```python
from build123d import *

# Parameters (mm, degrees)
F1_DEPTH = 16.002
F3_DEPTH = 16.002
F4_R     = 2.54


with BuildPart() as f1:
    # F0 (on Top) → F1 (new body)
    with BuildSketch(Plane.XY):
        with BuildLine():
            ThreePointArc((38.1, -7.874), (48.1578868556, -3.7078868556), (52.324, 6.35))
            Line((52.324, 6.35), (52.324, 38.1))
            Line((52.324, 38.1), (-14.224, 38.1))
            Line((-14.224, 38.1), (-14.224, 6.35))
            ThreePointArc((-14.224, 6.35), (-10.0578868556, -3.7078868556), (0, -7.874))
            Line((0, -7.874), (38.1, -7.874))
        make_face()
        with BuildLine():
            Line((38.1, 0), (0, 0))
            ThreePointArc((0, 0), (-6.35, 6.35), (0, 12.7))
            Line((0, 12.7), (38.1, 12.7))
            ThreePointArc((38.1, 12.7), (44.45, 6.35), (38.1, 0))
        make_face(mode=Mode.SUBTRACT)
    extrude(amount=F1_DEPTH)

    # F2 (on face) → F3 (join)
    with BuildSketch(Plane(origin=(0, 38.1, 0), x_dir=(-1, 0, 0), z_dir=(0, 1, 0))):
        with BuildLine():
            Line((26.924, 0), (26.924, 44.45))
            Line((26.924, 44.45), (20.574, 44.45))
            ThreePointArc((20.574, 44.45), (14.224, 38.1), (7.874, 44.45))
            Line((7.874, 44.45), (1.524, 44.45))
            Line((1.524, 44.45), (1.524, 0))
            Line((1.524, 0), (26.924, 0))
        make_face()
        with BuildLine():
            Line((20.574, 44.45), (26.924, 44.45))
            ThreePointArc((26.924, 44.45), (14.224, 57.15), (1.524, 44.45))
            Line((1.524, 44.45), (7.874, 44.45))
            ThreePointArc((7.874, 44.45), (14.224, 50.8), (20.574, 44.45))
        make_face()
        with BuildLine():
            Line((-39.624, 0), (-39.624, 44.45))
            Line((-39.624, 44.45), (-45.974, 44.45))
            ThreePointArc((-45.974, 44.45), (-52.324, 38.1), (-58.674, 44.45))
            Line((-58.674, 44.45), (-65.024, 44.45))
            Line((-65.024, 44.45), (-65.024, 0))
            Line((-65.024, 0), (-39.624, 0))
        make_face()
        with BuildLine():
            Line((-45.974, 44.45), (-39.624, 44.45))
            ThreePointArc((-39.624, 44.45), (-52.324, 57.15), (-65.024, 44.45))
            Line((-65.024, 44.45), (-58.674, 44.45))
            ThreePointArc((-58.674, 44.45), (-52.324, 50.8), (-45.974, 44.45))
        make_face()
    extrude(amount=-F3_DEPTH)

    # F4
    f4_edges = [f1.edges().sort_by_distance(p)[0] for p in [
        (52.324, 14.224, 16.002),
        (-10.057887, -3.707887, 16.002),
        (-14.224, 14.224, 16.002),
        (-7.874, 22.098, 16.002),
        (-1.524, 30.099, 16.002),
        (19.05, 38.1, 16.002),
        (39.624, 30.099, 16.002),
        (45.974, 22.098, 16.002),
        (48.157887, -3.707887, 16.002),
        (19.05, -7.874, 16.002),
        (44.45, 6.35, 16.002),
        (19.05, 12.7, 16.002),
        (19.05, 0, 16.002),
        (-6.35, 6.35, 16.002),
        (52.324, 22.098, 8.001),
        (52.324, 38.1, 57.15),
        (65.024, 38.1, 22.225),
        (39.624, 38.1, 30.226),
        (-1.524, 38.1, 30.226),
        (-14.224, 38.1, 57.15),
        (-26.924, 38.1, 22.225),
        (-14.224, 22.098, 8.001),
    ]]
    fillet(f4_edges, radius=F4_R)


solid = f1.part
```
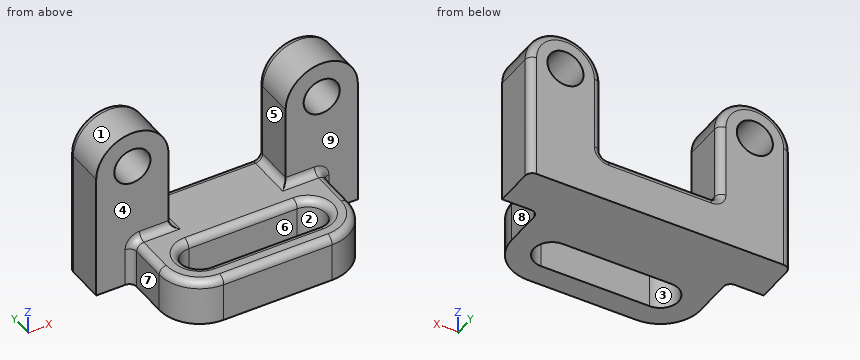
Design review of the part built by this model. Coordinates are the model's own, in mm. Face numbers are marked on the shaded views. A direction names the side the tool comes from. Coordinates: 2 decimals unless noted, no trailing zeros. Write each loop counter-clockwise with the first axis right and the second up, starting at its lowest first coordinate (ties: lowest second). Pieces come first, ordered by that corner, then holes.
1) Add section D-D (y = 21). Write out the cut boundary in (x, z).
2) Machinability: for the marked faces 5, 6, 7, 8 and 9, which of the approach directions +Z, -Z, +X, -X, +Y, -Y give a long, thin tool a straight path to every point of the face, cutting with its end or side? Answer none if there is none.
3) Add section A-A (z = 29). Write out the cut boundary in (x, y), plus the area to 3 significant figures.
4) Add section B-B (x = 9). Write out the cut boundary in (y, z), plus the area to 3 significant figures.
5) Mouldability with a two-part tool opening along Y and no side actions: class the marked faces 1, 2, 3 and 4 as +Y half, -Y half, draft (parallel to the pull), parting line (faces both ways), or undercut.
6) Insertion check: pin 1 (10.5 mm diameter, centred on y = 11, z = 4, fed in from +X); pin 2 (4 mm diameter, centred on x = -9, y = 22.5, fed in from -Z); pin 3 (12.5 mm diameter, centred on x = -15.5, z = 27, fed in from -Y); pin 4 (12.5 mm diameter, centred on x = 12, y = 10.5, fed in from +Z). Each pin has a flat end and moves straight along its axis. Give the tip position at first contact, or say it passes through.
7) To check wall thickness, follow L1, parallel to X at y = 33, z = 44; L2, parallel to Y at x = 38.5, z = 4; L3, parallel to X at y = 33.5, z = 19.5. State the ranges of each line that lie inside material, in increasing order.
8) Add section C-C (z = 9). Write out the cut boundary in (x, y).
Check result:
1. outline: (-14.67, 0) - (52.77, 0) - (52.77, 13.46) arc R2.99 ccw to (49.78, 16.45) - (38.53, 16.45) arc R2.54 cw to (37.08, 16) - (1.02, 16) arc R2.54 cw to (-0.43, 16.45) - (-11.68, 16.45) arc R2.99 ccw to (-14.67, 13.46) - close
2. face 5: +Z, +Y, -Y
2. face 6: +Z, -Z
2. face 7: +Z, -Z, -X, -Y
2. face 8: +Z, -Z, +X, -Y
2. face 9: +Z, +X, -Y
3. outline: (-26.92, 22.1) - (-1.52, 22.1) - (-1.52, 35.56) arc R2.54 ccw to (-4.06, 38.1) - (-24.38, 38.1) arc R2.54 ccw to (-26.92, 35.56) - close; (39.62, 22.1) - (65.02, 22.1) - (65.02, 35.56) arc R2.54 ccw to (62.48, 38.1) - (42.16, 38.1) arc R2.54 ccw to (39.62, 35.56) - close
3. area: 807 mm2
4. outline: (-7.87, 0) - (0, 0) - (0, 13.46) arc R2.54 ccw to (-2.54, 16) - (-5.33, 16) arc R2.54 ccw to (-7.87, 13.46) - close; (12.7, 0) - (38.1, 0) - (38.1, 13.46) arc R2.54 ccw to (35.56, 16) - (15.24, 16) arc R2.54 ccw to (12.7, 13.46) - close
4. area: 527 mm2
5. face 1: draft
5. face 2: undercut
5. face 3: undercut
5. face 4: -Y half
6. pin 1: stops at x = 52.32
6. pin 2: stops at z = 0
6. pin 3: stops at y = 22.1
6. pin 4: stops at z = 16
7. L1: x = -26.92 to -20.56, -7.89 to -1.52, 39.62 to 45.99, 58.66 to 65.02
7. L2: y = -7.87 to 0.01, 12.69 to 38.1
7. L3: x = -26.92 to -1.52, 39.62 to 65.02
8. outline: (-26.92, 22.1) - (-16.76, 22.1) arc R2.54 cw to (-14.22, 19.56) - (-14.22, 6.35) arc R14.22 ccw to (0, -7.87) - (38.1, -7.87) arc R14.22 ccw to (52.32, 6.35) - (52.32, 19.56) arc R2.54 cw to (54.86, 22.1) - (65.02, 22.1) - (65.02, 35.56) arc R2.54 ccw to (62.48, 38.1) - (-24.38, 38.1) arc R2.54 ccw to (-26.92, 35.56) - close; hole (0, 0) - (38.1, 0) arc R6.35 ccw to (38.1, 12.7) - (0, 12.7) arc R6.35 ccw to start
